Part model, mm, in its own coordinate system. A direction names the side the tool comes from. Give positions to 0.01 mm unless a question says otherwise; leave off trailing zeros. Order: outer loops, then holes, each group sorted by start corner. A loop starts at its lowest first (then second) coordinate and runs counter-clockwise, first axis right, second up. Notation, with made-up numbers: (21, 6) - (42, 6) arc R20 cw to (42, 11) - close; hole circle Ø6 at (31, 73.25). An arc over 180 degrees is marked (long way). Use a Markdown table: item, result. Add a question column.
from build123d import *

# Parameters (mm, degrees)
SKETCH_R        = 5.95
SKETCH_R_2      = 12.5
SKETCH_R_3      = 1.5
PAD_DEPTH       = 30
SKETCH001_W     = 42
SKETCH001_H     = 42
POCKET_DEPTH    = 7
SKETCH002_R     = 3
POCKET001_DEPTH = 3
SKETCH003_R     = 10.4
SKETCH003_R_2   = 5
SKETCH003_R_3   = 1.5
POCKET002_DEPTH = 60
SKETCH004_W     = 21
SKETCH004_H     = 21
POCKET003_DEPTH = 20
FILLET_R        = 1


with BuildPart() as part:
    # Sketch → Pad (new body)
    with BuildSketch(Plane.YZ):
        with BuildLine():
            Line((-15, -46.568569), (-15, -64.955837))
            ThreePointArc((-24.667572, -74.62341), (-17.831566, -71.791843), (-15, -64.955837))
            Line((-24.667572, -74.62341), (-30, -74.62341))
            Line((-30, -74.62341), (-30, -124.62341))
            Line((-30, -124.62341), (30, -124.62341))
            Line((30, -124.62341), (30, -74.62341))
            Line((30, -74.62341), (25.245382, -74.62341))
            ThreePointArc((15, -64.378028), (18.000803, -71.622607), (25.245382, -74.62341))
            Line((15, -46.619995), (15, -64.378028))
            ThreePointArc((15.724488, -43.551034), (15.183577, -45.043337), (15, -46.619995))
            Line((24.011209, -26.977709), (15.724488, -43.551034))
            ThreePointArc((24.011209, -26.977709), (24.749504, -24.940849), (25.00007, -22.788851))
            Line((25.00007, 22.051522), (25.00007, -22.788851))
            ThreePointArc((25.00007, 22.051522), (24.055257, 25.311646), (21.513639, 27.561371))
            Line((21.513639, 27.561371), (-6.871688, 41.010422))
            ThreePointArc((-6.871688, 41.010422), (-13.83329, 41.395689), (-19.079268, 36.803082))
            Line((-19.079268, 36.803082), (-24.067049, 26.849336))
            ThreePointArc((-24.067049, 26.849336), (-24.759326, 24.943331), (-24.994291, 22.929158))
            Line((-24.994291, -22.260199), (-24.994291, 22.929158))
            ThreePointArc((-24.994291, -22.260199), (-24.682525, -24.93782), (-23.763909, -27.472183))
            Line((-23.763909, -27.472183), (-15.701485, -43.597029))
            ThreePointArc((-15, -46.568569), (-15.177749, -45.041961), (-15.701485, -43.597029))
        make_face()
        with Locations((0, 24.5)):
            Circle(SKETCH_R, mode=Mode.SUBTRACT)
        with Locations((0, -24.5)):
            Circle(SKETCH_R, mode=Mode.SUBTRACT)
        Circle(SKETCH_R_2, mode=Mode.SUBTRACT)
        with Locations((-15, 15)):
            Circle(SKETCH_R_3, mode=Mode.SUBTRACT)
        with Locations((-15, -15)):
            Circle(SKETCH_R_3, mode=Mode.SUBTRACT)
        with Locations((15, -15)):
            Circle(SKETCH_R_3, mode=Mode.SUBTRACT)
        with Locations((15, 15)):
            Circle(SKETCH_R_3, mode=Mode.SUBTRACT)
    extrude(amount=PAD_DEPTH)

    # Sketch001 (on Face30 of Pad) → Pocket (cut)
    with BuildSketch(Plane(origin=(0, 0, 0), x_dir=(0, 1, 0), z_dir=(-1, 0, 0))):
        Rectangle(SKETCH001_W, SKETCH001_H)
    extrude(amount=-POCKET_DEPTH, mode=Mode.SUBTRACT)

    # Sketch002 (on Face5 of Pocket) → Pocket001 (cut)
    with BuildSketch(Plane.YZ.offset(30)):
        with Locations((-15, 15)):
            Circle(SKETCH002_R)
        with Locations((15, 15)):
            Circle(SKETCH002_R)
        with Locations((-15, -15)):
            Circle(SKETCH002_R)
        with Locations((15, -15)):
            Circle(SKETCH002_R)
    extrude(amount=-POCKET001_DEPTH, mode=Mode.SUBTRACT)

    # Sketch003 (on Face9 of Pocket001) → Pocket002 (cut)
    with BuildSketch(Plane(origin=(0, -30, 0), x_dir=(0, 0, -1), z_dir=(0, -1, 0))):
        with Locations((89.62341, 15)):
            Circle(SKETCH003_R)
        with Locations((111.62341, 15)):
            Circle(SKETCH003_R_2)
        with Locations((111.62341, 22.5)):
            Circle(SKETCH003_R_3)
        with Locations((104.12341, 15)):
            Circle(SKETCH003_R_3)
        with Locations((119.12341, 15)):
            Circle(SKETCH003_R_3)
        with Locations((111.62341, 7.5)):
            Circle(SKETCH003_R_3)
    extrude(amount=-POCKET002_DEPTH, mode=Mode.SUBTRACT)

    # Sketch004 (on Face9 of Pocket002) → Pocket003 (cut)
    with BuildSketch(Plane(origin=(0, -30, 0), x_dir=(0, 0, -1), z_dir=(0, -1, 0))):
        with Locations((111.62341, 15)):
            Rectangle(SKETCH004_W, SKETCH004_H)
    extrude(amount=-POCKET003_DEPTH, mode=Mode.SUBTRACT)

    # Fillet
    fillet_edges = [part.edges().sort_by_distance(p)[0] for p in [
        (0, -30, -99.62341),
        (15, -24.667572, -74.62341),
        (15, -30, -74.62341),
        (0, -27.333786, -74.62341),
        (30, -27.333786, -74.62341),
        (30, -30, -99.62341),
        (15, 30, -74.62341),
        (0, 30, -99.62341),
        (30, 30, -99.62341),
    ]]
    fillet(fillet_edges, radius=FILLET_R)


solid = part.part
1. Tool access for faces 5 (the face through (28.5, 12.6, 13.2)), 6 (the face through (15, -24.994, 0)), 7 (the face through (14.8, 17.92, -71.54)), 8 (the face through (25.5, -20, -111)): list every direction of +Z, -Z, +X, -X, +Y, -Y with a clear straight run to the whole face (end or side of a thin tool).
2. Cut at B-B (x = 15). State how many separate pieces and enclosed holes the cut face has, plus the area to 3 significant figures.
3. Pin check, flat tips, straight feed: P1, Ø7.5, axis at x = 3.5, z = 1.5, coming from the +Y side; P2, Ø5, axis at x = 25.5, y = -12.5, coming from the +Z side; P3, Ø3, axis at y = -15, z = 16, coming from the +X side; P4, Ø15, axis at y = 0, z = 0, coming from the +X side. Stop position of each tip, or through.
4. Cut at C-C (z = -96). Write the cut outline in (x, y).
5. Drill centre lines: probe 1 along Y at (x, z) = (22, -15); probe 2 along Z at (x, y) = (10.5, 11.5); probe 3 along Y at (x, z) = (19, 16). Where is each one in solid material? Low to high. Write a range as [from, to].
6. Cut at A-A (z = 0). Write the cut outline in (x, y), plus the area to 3 significant figures.
7. Mould opens along X. For faces 1 (the face through (0.285, -19.407, -35.513)), 2 (the face through (17.5, -10, -106.8)), 3 (the face through (29.715, 6.994, 34.108)), 4 (the face through (16.86, -16.5, -14.93)) say: released by +X, released by -X, zero draft, split by the parting line, or undercut.
Responses:
| question | item | result |
|---|---|---|
| 1 | face 5 | +X |
| 1 | face 6 | +Z, +X, -X, -Y |
| 1 | face 7 | +X, -X, +Y |
| 1 | face 8 | -Y |
| 2 | separate pieces | 5 |
| 2 | enclosed holes | 7 |
| 2 | area | 4,680 mm² |
| 3 | P1 | stops at y = 25 |
| 3 | P2 | stops at z = 41.9 |
| 3 | P3 | stops at x = 27 |
| 3 | P4 | passes through |
| 4 | outline | (0, -29) arc R1 ccw to (1, -30) - (6.78, -30) - (6.78, 30) - (1, 30) arc R1 ccw to (0, 29) - close; (23.22, -30) - (29, -30) arc R1 ccw to (30, -29) - (30, 29) arc R1 ccw to (29, 30) - (23.22, 30) - close |
| 5 | probe 1 | y = [-24.99, -16.5], [-13.5, 13.5], [16.5, 25] |
| 5 | probe 2 | z = [-124.62, -113.8], [-109.44, -99], [-80.25, -4.9], [4.9, 32.31] |
| 5 | probe 3 | y = [-24.99, -16.12], [-13.88, 13.88], [16.12, 25] |
| 6 | outline | (0, -23.99) arc R1 ccw to (1, -24.99) - (29, -24.99) arc R1 ccw to (30, -23.99) - (30, -12.5) - (7, -12.5) - (7, -21) - (0, -21) - close; (0, 21) - (7, 21) - (7, 12.5) - (30, 12.5) - (30, 24) arc R1 ccw to (29, 25) - (1, 25) arc R1 ccw to (0, 24) - close |
| 6 | area | 630 mm² |
| 7 | face 1 | released by -X |
| 7 | face 2 | undercut |
| 7 | face 3 | released by +X |
| 7 | face 4 | zero draft |
